Geometry: see drawing. Coordinates: mm, zero at the bounding-box minimum. A direction names the side the tool comes from. Round coordinates to 2 decimals unless told otherwise and drop trailing zeros. Loops run counter-clockwise (first coordinate to the right, second up) from the corner with the lowest first, then second, coordinate; pieces in that order, holes last.
(1) Cut plane D-D, the plane x = 17.5. Output: boundary loops of the cut face in (y, z), and give its area (3 significant figures).
(2) First-contact query: pin 1 Ø5 at (y, z) = (31.5, 24) entering from -X; pin 2 Ø4.5 at (x, z) = (39, 39) entering from +Y; pin 3 Ø1 at (y, z) = (93, 13.5) entering from -X. Flat tips, straight axial feed; report the tip coordinate or a pass-through.
(3) Cut plane B-B, the plane x = 34. Output: boundary loops of the cut face in (y, z).
(4) Cut plane C-C, the plane y = 126.5. Output: boundary loops of the cut face in (x, z), and give its area (4 significant figures).
(5) Access query for the marked faces 1, 2, 3 and 4. Directions: +Z, -Z, +X, -X, +Y, -Y. A direction counts if a zero-diameter tool reaches every point of the face in a straight line with its end or side. Return the directions, or none.
(6) Line query: line 1 (X direction, y = 67, z = 3.5); line 2 (Y direction, x = 16, z = 14.5); line 3 (Y direction, x = 38, z = 3). Output: solid intervals per line, ascending.
(7) Cut plane A-A, the plane z = 20.25. Output: boundary loops of the cut face in (x, y), and give its area (3 significant figures).
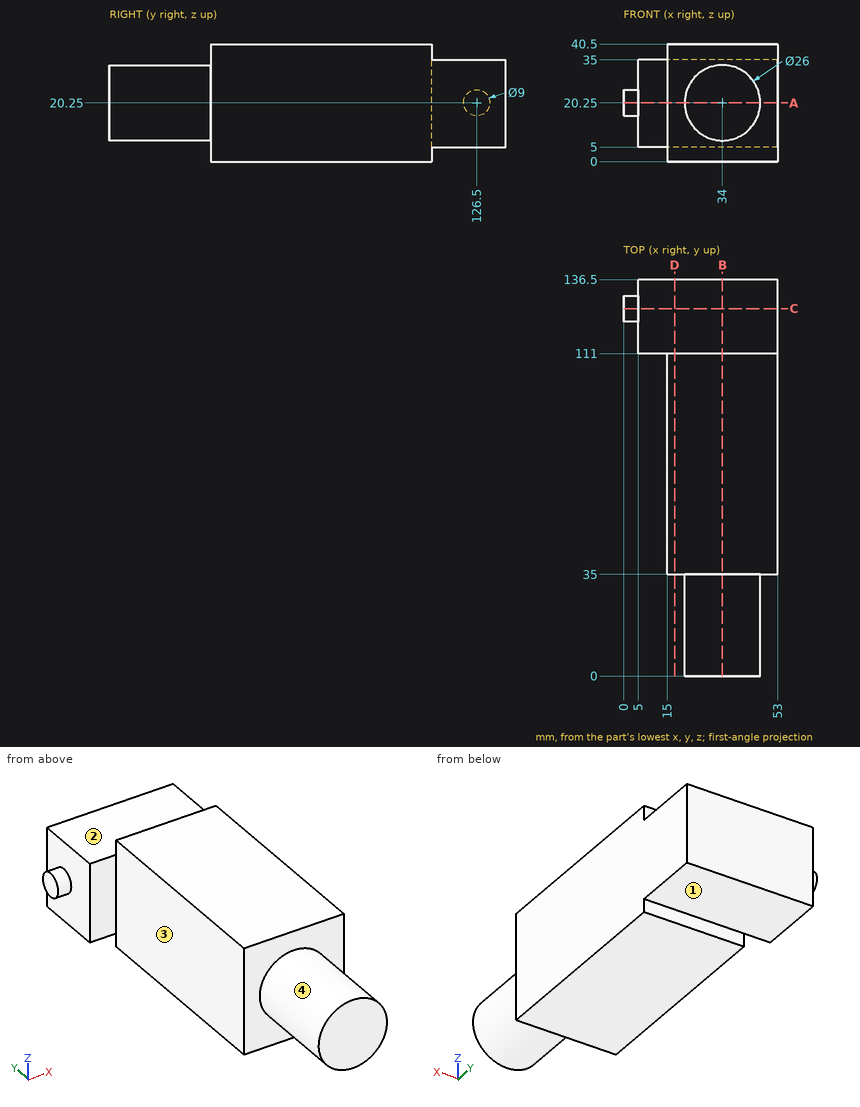
Reported:
1. outline: (35, 0) - (111, 0) - (111, 5) - (136.5, 5) - (136.5, 35) - (111, 35) - (111, 40.5) - (35, 40.5) - close
1. area: 3,840 mm2
2. pin 1: stops at x = 21.06
2. pin 2: stops at y = 111
2. pin 3: stops at x = 15
3. outline: (0, 7.25) - (35, 7.25) - (35, 0) - (111, 0) - (111, 5) - (136.5, 5) - (136.5, 35) - (111, 35) - (111, 40.5) - (35, 40.5) - (35, 33.25) - (0, 33.25) - close
4. outline: (0, 15.75) - (5, 15.75) - (5, 5) - (53, 5) - (53, 35) - (5, 35) - (5, 24.75) - (0, 24.75) - close
4. area: 1,485 mm2
5. face 1: -Z, +X, -X, +Y
5. face 2: +Z, +X, -X, +Y
5. face 3: +Z, -Z, -X, -Y
5. face 4: -Y
6. line 1: x = 15 to 53
6. line 2: y = 35 to 136.5
6. line 3: y = 35 to 111
7. outline: (0, 122) - (5, 122) - (5, 111) - (15, 111) - (15, 35) - (21, 35) - (21, 0) - (47, 0) - (47, 35) - (53, 35) - (53, 136.5) - (5, 136.5) - (5, 131) - (0, 131) - close
7. area: 5,070 mm2
